Here's how the part is built. I have some questions about the finished solid (model axes, mm). A direction names the side the tool comes from. Round coordinates to 2 decimals unless told otherwise and drop trailing zeros. Write each loop counter-clockwise with the first axis right and the second up, starting at its lowest first coordinate (ties: lowest second). Pieces come first, ordered by that corner, then holes. Notation, with made-up numbers: (80.25, 7) -> (125.25, 7) arc R25 ccw to (125.25, 20) -> close; hole circle Ø9 at (48.5, 85.5). An arc over 180 degrees is marked (long way). Answer in a Markdown table with one row per item. Add a question column.
from build123d import *

# Parameters (mm, degrees)
CROQUIS3_W              = 26.7
CROQUIS3_H              = 26.7
CROQUIS3_W_2            = 4
CROQUIS3_H_2            = 25.7
SALIENTE_EXTRUIR1_DEPTH = 50
CORTAR_EXTRUIR14_REACH  = 74.827
REDONDEO2_R             = 2.5
CORTAR_EXTRUIR19_REACH  = 75.253
CROQUIS18_W             = 7
CROQUIS18_H             = 42
CROQUIS19_W             = 4
CROQUIS19_H             = 2
CROQUIS19_W_2           = 3
CROQUIS19_H_2           = 20
SALIENTE_EXTRUIR3_DEPTH = 50
CORTAR_EXTRUIR20_REACH  = 80.262
CROQUIS20_W             = 44
CROQUIS20_H             = 3.6
CORTAR_EXTRUIR21_REACH  = 89.71
REDONDEO6_R             = 3
REDONDEO9_R             = 1.3
CORTAR_EXTRUIR22_REACH  = 75.253
CROQUIS22_W             = 7
CROQUIS22_H             = 42
REDONDEO10_R            = 6.5


with BuildPart() as part:
    # Croquis3 → Saliente-Extruir1 (new body)
    with BuildSketch(Plane.XY):
        Polygon((-43.857247249, 6.480922369), (-6.157247249, 6.480922369), (-6.157247249, 37.180922369), (-27.007247249, 37.180922369), (-43.857247249, 37.180922369), align=None)
        with Locations((-28.507247249, 21.830922369)):
            Rectangle(CROQUIS3_W, CROQUIS3_H, mode=Mode.SUBTRACT)
        with Locations((-11.157247249, 22.330922369)):
            Rectangle(CROQUIS3_W_2, CROQUIS3_H_2, mode=Mode.SUBTRACT)
    extrude(amount=SALIENTE_EXTRUIR1_DEPTH)

    # Cortar-Extruir14: up to this face of the body (flat: up to its plane)
    cortar_extruir14_end = Plane(part.part.faces().sort_by_distance((-15.157247249, 21.830922369, 25))[0])
    # Croquis14 → Cortar-Extruir14 (cut, up to the picked face)
    with BuildSketch(Plane(origin=(-6.157247249, 0, 0), x_dir=(0, 0, -1), z_dir=(1, 0, 0)), mode=Mode.PRIVATE) as cortar_extruir14_sk1:
        Polygon((-2.979356026, 22.330922369), (-2.979356026, 19.830922369), (-47.020643974, 19.830922369), (-47.020643974, 22.330922369), (-47.020643974, 24.830922369), (-2.979356026, 24.830922369), align=None)
    cortar_extruir14_tool1 = split(extrude(cortar_extruir14_sk1.sketch, amount=-CORTAR_EXTRUIR14_REACH, mode=Mode.PRIVATE), bisect_by=cortar_extruir14_end, keep=Keep.BOTH, mode=Mode.PRIVATE)
    add(cortar_extruir14_tool1.solids().sort_by(Axis((-6.157247, 22.330922, 25), (-1, 0, 0)))[0], mode=Mode.SUBTRACT)

    # Redondeo2
    redondeo2_edges = [part.edges().sort_by_distance(p)[0] for p in [
        (-14.157247249, 24.830922369, 2.979356026),
        (-7.657247249, 24.830922369, 2.979356026),
        (-7.657247249, 19.830922369, 2.979356026),
        (-14.157247249, 19.830922369, 2.979356026),
        (-14.157247249, 24.830922369, 47.020643974),
        (-7.657247249, 24.830922369, 47.020643974),
        (-7.657247249, 19.830922369, 47.020643974),
        (-14.157247249, 19.830922369, 47.020643974),
    ]]
    fillet(redondeo2_edges, radius=REDONDEO2_R - 0.0001)  # a hair under: the kernel refuses the full size

    # Croquis18 → Cortar-Extruir19 (cut, up to next)
    with BuildSketch(Plane(origin=(0, 37.180922369, 0), x_dir=(1, 0, 0), z_dir=(0, 1, 0)), mode=Mode.PRIVATE) as cortar_extruir19_sk1:
        with Locations((-28.507247249, -25)):
            Rectangle(CROQUIS18_W, CROQUIS18_H)
    cortar_extruir19_tool1 = extrude(cortar_extruir19_sk1.sketch, amount=-CORTAR_EXTRUIR19_REACH, mode=Mode.PRIVATE) & part.part
    add(cortar_extruir19_tool1.solids().sort_by_distance((-28.507247, 37.180922, 25))[0], mode=Mode.SUBTRACT)

    # Croquis19 → Saliente-Extruir3 (add)
    with BuildSketch(Plane(origin=(0, 0, 0), x_dir=(-1, 0, 0), z_dir=(0, 0, -1))):
        with Locations((11.157247249, 16.330922369)):
            Rectangle(CROQUIS19_W, CROQUIS19_H)
        with Locations((11.157247249, 28.330922369)):
            Rectangle(CROQUIS19_W, CROQUIS19_H)
        with Locations((23.507247249, 47.180922369)):
            Rectangle(CROQUIS19_W_2, CROQUIS19_H_2)
    extrude(amount=-SALIENTE_EXTRUIR3_DEPTH)

    # Croquis20 → Cortar-Extruir20 (cut, up to next)
    with BuildSketch(Plane.ZY.offset(25.007247249), mode=Mode.PRIVATE) as cortar_extruir20_sk1:
        with Locations((25, 46.180922369)):
            Rectangle(CROQUIS20_W, CROQUIS20_H)
    cortar_extruir20_tool1 = extrude(cortar_extruir20_sk1.sketch, amount=-CORTAR_EXTRUIR20_REACH, mode=Mode.PRIVATE) & part.part
    add(cortar_extruir20_tool1.solids().sort_by_distance((-25.007247, 46.180922, 25))[0], mode=Mode.SUBTRACT)

    # Croquis21 → Cortar-Extruir21 (cut, up to next)
    with BuildSketch(Plane(origin=(0, 0, 0), x_dir=(-1, 0, 0), z_dir=(0, 0, -1)), mode=Mode.PRIVATE) as cortar_extruir21_sk1:
        Polygon((13.157247249, 35.180922369), (13.157247249, 37.180922369), (6.157247249, 37.180922369), (6.157247249, 29.330922369), (9.157247249, 29.330922369), (9.157247249, 35.180922369), align=None)
    cortar_extruir21_tool1 = extrude(cortar_extruir21_sk1.sketch, amount=-CORTAR_EXTRUIR21_REACH, mode=Mode.PRIVATE) & part.part
    # Croquis21 → Cortar-Extruir21 (cut, up to next)
    with BuildSketch(Plane(origin=(0, 0, 0), x_dir=(-1, 0, 0), z_dir=(0, 0, -1)), mode=Mode.PRIVATE) as cortar_extruir21_sk2:
        Polygon((6.157247249, 9.480922369), (6.157247249, 15.330922369), (9.157247249, 15.330922369), (9.157247249, 9.480922369), (13.157247249, 9.480922369), (13.157247249, 6.480922369), (6.157247249, 6.480922369), align=None)
    cortar_extruir21_tool2 = extrude(cortar_extruir21_sk2.sketch, amount=-CORTAR_EXTRUIR21_REACH, mode=Mode.PRIVATE) & part.part
    add(cortar_extruir21_tool1.solids().sort_by_distance((-8.544727, 33.997602, 0))[0], mode=Mode.SUBTRACT)
    add(cortar_extruir21_tool2.solids().sort_by_distance((-8.746741, 9.995417, 0))[0], mode=Mode.SUBTRACT)

    # Redondeo6
    redondeo6_edges = [part.edges().sort_by_distance(p)[0] for p in [
        (-13.157247249, 15.330922369, 25),
        (-13.157247249, 29.330922369, 25),
    ]]
    fillet(redondeo6_edges, radius=REDONDEO6_R)

    # Redondeo9
    redondeo9_edges = [part.edges().sort_by_distance(p)[0] for p in [
        (-23.507247249, 47.980922369, 3),
        (-23.507247249, 47.980922369, 47),
        (-23.507247249, 44.380922369, 47),
        (-23.507247249, 44.380922369, 3),
    ]]
    fillet(redondeo9_edges, radius=REDONDEO9_R)

    # Croquis22 → Cortar-Extruir22 (cut, up to next)
    with BuildSketch(Plane(origin=(0, 37.180922369, 0), x_dir=(1, 0, 0), z_dir=(0, 1, 0)), mode=Mode.PRIVATE) as cortar_extruir22_sk1:
        with Locations((-35.507247249, -25)):
            Rectangle(CROQUIS22_W, CROQUIS22_H)
    cortar_extruir22_tool1 = extrude(cortar_extruir22_sk1.sketch, amount=-CORTAR_EXTRUIR22_REACH, mode=Mode.PRIVATE) & part.part
    add(cortar_extruir22_tool1.solids().sort_by_distance((-35.507247, 37.180922, 25))[0], mode=Mode.SUBTRACT)

    # Redondeo10
    redondeo10_edges = [part.edges().sort_by_distance(p)[0] for p in [
        (-25.007247249, 36.180922369, 46),
        (-25.007247249, 36.180922369, 4),
        (-39.007247249, 36.180922369, 4),
        (-39.007247249, 36.180922369, 46),
    ]]
    fillet(redondeo10_edges, radius=REDONDEO10_R)


solid = part.part
Item 1: On a 3-axis mill with a long thin cutter (end or side, diameter ignored), from which of +Z, -Z, +X, -X, +Y, -Y can I reach the whole of each face in a straight line? I mean faces 1 (the flat face through (-8, 15.331, 25)), 2 (the flat face through (-11, 27.331, 25)), 3 (the cylindrical face through (-14.171, 24.118, 3.731)), 4 (the flat face through (-8, 29.331, 25)), 5 (the flat face through (-24, 47.981, 25)). Say none if no direction works.
Item 2: If we mould it in two halves opening along X, with no side actions, what happens to faces 6 (the cylindrical face through (-37.1, 36.2, 44.1)), 7 (the flat face through (-22.007, 49, 25)), 8 (the cylindrical face through (-7.678, 20.544, 46.269))? For each: pulls with the +X half, pulls with the -X half, needs draft (parallel to the pull), parting line crosses it, or undercut.
Item 3: If we section it at A-A on x = -19.5: Please give me the cut outline in (y, z), then the cut area to 3 significant figures.
Item 4: If we section it at C-C on x = -36.5: Please give me the cut outline in (y, z), then the cut area to 3 significant figures.
Item 5: For P1, Ø10, axis at x = -23, y = 13, coming from the -Z side; P2, Ø2.5, axis at x = -8, z = 21.5, coming from the +Y side; P3, Ø3, axis at x = -10.5, z = 32.5, coming from the +Y side; P4, Ø1, axis at y = 36.5, z = 32, coming from the +X side, each with a flat end and sliding along its axis, tell me the tip position at first contact or that it passes through.
Item 6: I need wall thicknesses on line 1 along X through (y, z) = (19, 25); line 2 along Y through (x, z) = (-23.5, 44.5); line 3 along Y through (x, z) = (-9.5, 42). Which ranges of each line are inside material? Lowest first, please. Write a range as from..to.
Item 7: If we section it at B-B on y = 11: Please give me the cut outline in (x, z).
Item 8: If we section it at D-D on z = 30: Give the number of separate pieces and of enclosed holes in the cut face, then the cut area to 3 significant figures.
Results list:
| question | item | result |
|---|---|---|
| 1 | face 1 | +Z, -Z, +X, -Y |
| 1 | face 2 | +Z, -Z |
| 1 | face 3 | +X |
| 1 | face 4 | +Z, -Z, +X, +Y |
| 1 | face 5 | +X, -X |
| 2 | face 6 | undercut |
| 2 | face 7 | pulls with the +X half |
| 2 | face 8 | needs draft |
| 3 | outline | (6.48, 0) -> (8.48, 0) -> (8.48, 50) -> (6.48, 50) -> close; (35.18, 0) -> (37.18, 0) -> (37.18, 50) -> (35.18, 50) -> close |
| 3 | area | 200 mm² |
| 4 | outline | (6.48, 0) -> (8.48, 0) -> (8.48, 50) -> (6.48, 50) -> close; (35.18, 0) -> (37.18, 0) -> (37.18, 5.37) -> (35.18, 5.37) -> close; (35.18, 44.63) -> (37.18, 44.63) -> (37.18, 50) -> (35.18, 50) -> close |
| 4 | area | 121 mm² |
| 5 | P1 | z = 0 |
| 5 | P2 | y = 29.33 |
| 5 | P3 | y = 29.96 |
| 5 | P4 | x = -13.16 |
| 6 | line 1 | -43.86..-41.86, -15.16..-13.16, -9.16..-6.16 |
| 6 | line 2 | 6.48..8.48, 35.18..44.38, 47.98..57.18 |
| 6 | line 3 | 15.33..17.33, 27.33..29.33 |
| 7 | outline | (-43.86, 0) -> (-41.86, 0) -> (-41.86, 50) -> (-43.86, 50) -> close; (-15.16, 0) -> (-13.16, 0) -> (-13.16, 50) -> (-15.16, 50) -> close |
| 8 | separate pieces | 3 |
| 8 | enclosed holes | 0 |
| 8 | area | 288 mm² |
